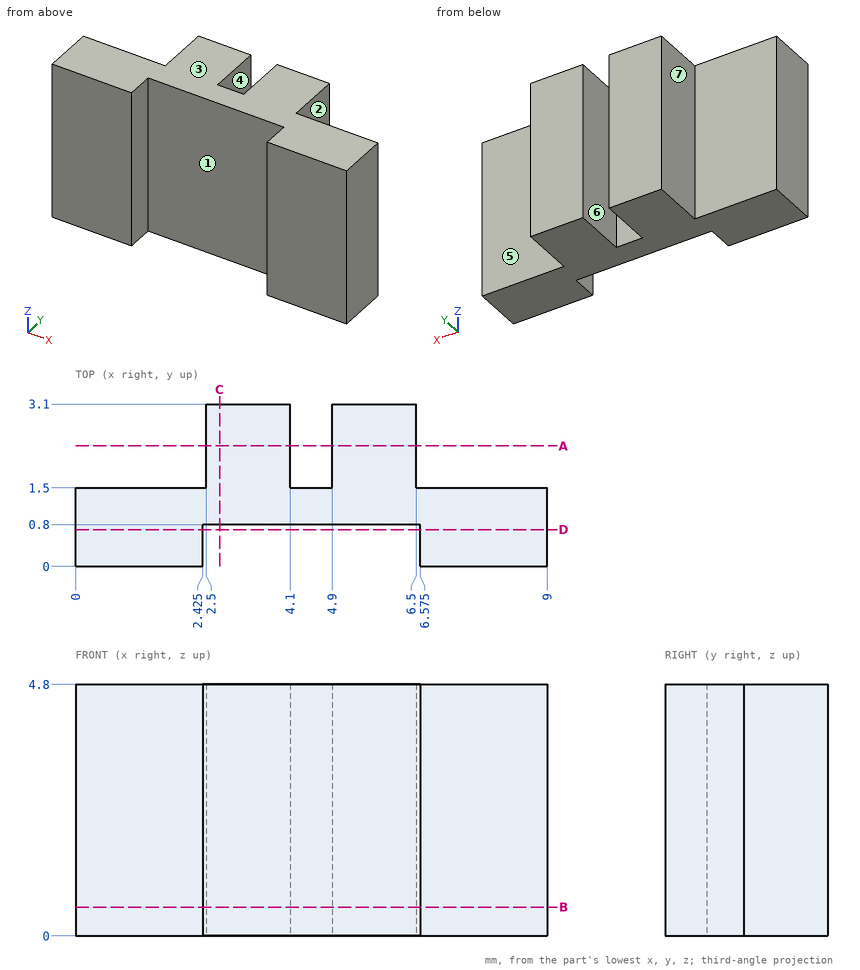
The drawing under review shows one solid part. Ordinate dimensions are in mm from its lowest x, y, z. A direction names the side the tool comes from. Round coordinates to 2 decimals unless told otherwise and drop trailing zeros. Loops run counter-clockwise (first coordinate to the right, second up) from the corner with the lowest first, then second, coordinate; pieces in that order, holes last. Notation, with made-up numbers: (28.25, 16) - (68.25, 16) arc R18 ccw to (68.25, 37) - close; hole circle Ø10 at (10.25, 36.5). An arc over 180 degrees is marked (long way). Use a Markdown table: item, result. Add a question column.
Q1. Add section A-A (y = 2.3). State the section outline as (x, z) points.
Q2. Add section B-B (z = 0.55). State the section outline as (x, y) points (3 decimals), plus the area to 3 significant figures.
Q3. Machinability: for the marked faces 5, 6 and 7, which of the approach directions +Z, -Z, +X, -X, +Y, -Y give a long, thin tool a straight path to every point of the face, cutting with its end or side? Answer none if there is none.
Q4. The part is to be moulded in two halves that separate along X. For the marked faces 1, 2, 3 and 4, say which applies: pulls with the +X half, pulls with the -X half, needs draft (parallel to the pull), parting line crosses it, or undercut.
Q5. Add section C-C (x = 2.75). State the section outline as (y, z) points, plus the area to 3 significant figures.
Q6. Add section D-D (y = 0.7). State the section outline as (x, z) points (3 decimals).
Q7. For probe 1 along X at (y, z) = (0.65, 3.45) (3 decimals); probe 2 along X at (y, z) = (2.2, 1.2); probe 3 along Y at (x, z) = (3.75, 4.45), list the stretches that pass through material, from the lowest coordinate up.
Q8. Insertion check: pin 1 Ø0.8 at (y, z) = (2.5, 1.5) entering from +X; pin 2 Ø1.3 at (y, z) = (2.5, 3) entering from -X. Each pin has a flat end and moves straight along its axis. Give the tip position at first contact, or say it passes through.
Worked answers:
| question | item | result |
|---|---|---|
| 1 | outline | (2.5, 0) - (4.1, 0) - (4.1, 4.8) - (2.5, 4.8) - close; (4.9, 0) - (6.5, 0) - (6.5, 4.8) - (4.9, 4.8) - close |
| 2 | outline | (0, 0) - (2.425, 0) - (2.425, 0.8) - (6.575, 0.8) - (6.575, 0) - (9, 0) - (9, 1.5) - (6.5, 1.5) - (6.5, 3.1) - (4.9, 3.1) - (4.9, 1.5) - (4.1, 1.5) - (4.1, 3.1) - (2.5, 3.1) - (2.5, 1.5) - (0, 1.5) - close |
| 2 | area | 15.3 mm² |
| 3 | face 5 | +Z, -Z, +X, +Y |
| 3 | face 6 | +Z, -Z, +Y |
| 3 | face 7 | +Z, -Z, -X, +Y |
| 4 | face 1 | undercut |
| 4 | face 2 | pulls with the +X half |
| 4 | face 3 | needs draft |
| 4 | face 4 | undercut |
| 5 | outline | (0.8, 0) - (3.1, 0) - (3.1, 4.8) - (0.8, 4.8) - close |
| 5 | area | 11.0 mm² |
| 6 | outline | (0, 0) - (2.425, 0) - (2.425, 4.8) - (0, 4.8) - close; (6.575, 0) - (9, 0) - (9, 4.8) - (6.575, 4.8) - close |
| 7 | probe 1 | 0 to 2.425, 6.575 to 9 |
| 7 | probe 2 | 2.5 to 4.1, 4.9 to 6.5 |
| 7 | probe 3 | 0.8 to 3.1 |
| 8 | pin 1 | x = 6.5 |
| 8 | pin 2 | x = 2.5 |
